Source: CAD feature listing. Evaluate the final solid. Frame: model axes, mm. A direction names the side the tool comes from. Give positions to 0.01 mm unless a question says otherwise; leave off trailing zeros. Order: outer loops, then holes, each group sorted by start corner. A loop starts at its lowest first (then second) coordinate and runs counter-clockwise, first axis right, second up.
from build123d import *

# Parameters (mm, degrees)
F3_DEPTH = 0.3
F4_R     = 1.5
F5_DEPTH = 4.5
F6_R     = 0.5


with BuildPart() as f3:
    # F2 (on Top) → F3 (new body)
    with BuildSketch(Plane.XY):
        with BuildLine():
            ThreePointArc((21.9341482237, -0.1564722617), (21.9660226591, 0), (21.9341482237, 0.1564722617))
            ThreePointArc((21.9341482237, 0.1564722617), (0, 14.6666666667), (-21.9341482237, 0.1564722617))
            ThreePointArc((-21.9341482237, 0.1564722617), (-21.9660226591, 0), (-21.9341482237, -0.1564722617))
            ThreePointArc((-21.9341482237, -0.1564722617), (0, -14.6666666667), (21.9341482237, -0.1564722617))
        make_face()
    extrude(amount=F3_DEPTH)

    # F4 (on face) → F5 (join)
    with BuildSketch(Plane.XY.offset(0.3)):
        with Locations((-5, 0)):
            Circle(F4_R)
        with Locations((5, 0)):
            Circle(F4_R)
    extrude(amount=F5_DEPTH)

    # F6
    f6_edges = [f3.edges().sort_by_distance(p)[0] for p in [
        (-6.5, 0, 4.8),
        (3.5, 0, 4.8),
    ]]
    fillet(f6_edges, radius=F6_R)


solid = f3.part
1) Section query A-A on z = 1. Output: boundary loops of the cut face in (x, y).
Checks:
outline: circle Ø3 at (-5, 0); circle Ø3 at (5, 0)
2) Section query D-D on x = -11.5. Output: boundary loops of the cut face in (y, z), and give its area (3 significant figures).
Checks:
outline: (-11.71, 0) - (11.71, 0) - (11.71, 0.3) - (-11.71, 0.3) - close
area: 7.03 mm2
3) First-contact query: pin 1 Ø14.5 at (x, y) = (0, 1) entering from +Z; pin 2 Ø1 at (x, z) = (-5, 3) entering from +Y. Flat tips, straight axial feed; report the tip coordinate or a pass-through.
Checks:
pin 1: stops at z = 4.8
pin 2: stops at y = 1.5
4) Ray query, L1, parallel to Z at x = -14.5, y = -6.5; L2, parallel to Y at x = -4, z = 2.45. Return the intervals inside material, ascending.
Checks:
L1: z = 0 to 0.3
L2: y = -1.12 to 1.12
5) Section query B-B on x = -5. Output: boundary loops of the cut face in (y, z).
Checks:
outline: (-14.14, 0) - (14.14, 0) - (14.14, 0.3) - (1.5, 0.3) - (1.5, 4.3) arc R0.5 ccw to (1, 4.8) - (-1, 4.8) arc R0.5 ccw to (-1.5, 4.3) - (-1.5, 0.3) - (-14.14, 0.3) - close
6) Pull-direction query (X, two-part tool) for faces 3 (the face through (5, 0, 4.8)), 4 (the face through (6.386, -0.575, 2.272)); classes: +X half, -X half, draft (parallel to the pull), parting line (faces both ways), or undercut.
Checks:
face 3: draft
face 4: undercut
7) Section query C-C on y = -8.5. Output: boundary loops of the cut face in (x, z), and give its area (3 significant figures).
Checks:
outline: (-16, 0) - (16, 0) - (16, 0.3) - (-16, 0.3) - close
area: 9.60 mm2
8) Reachability of faces 1 (the face through (0, 0, 0)), 2 (the face through (-6.2, -0.9, 2.3)) from +Z, -Z, +X, -X, +Y, -Y: full face, straight path, thin tool, end or side. Return the list, or none.
Checks:
face 1: -Z, +X, -X, +Y, -Y
face 2: +Z
